from build123d import *

# Parameters (mm, degrees)
FILLET1_R = 5


with BuildPart() as part:
    # Sketch1 → Revolve1 (revolve)
    with BuildSketch(Plane.XY):
        Polygon((16, 0), (9.5, 24.258330249), (9.5, 29.258330249), (18, 37.758330249), (18, 170), (22, 170), (22, 21.6), (20.5, 21.6), (20.5, 18.8), (22, 18.8), (22, 14.8), (20.5, 14.8), (20.5, 12), (22, 12), (22, 4), (19, 4), (19, 0), align=None)
    revolve(axis=Axis((0, 0, 0), (0, 1, 0)))

    # Fillet1
    fillet1_edges = [part.edges().sort_by_distance(p)[0] for p in [
        (-9.5, 29.258330249, 0),
        (-9.5, 24.258330249, 0),
    ]]
    fillet(fillet1_edges, radius=FILLET1_R)


solid = part.part
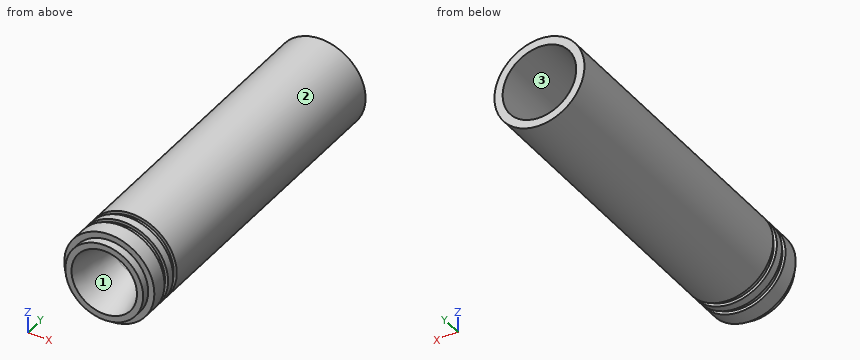
Verification items for the finished model (mm, model axes). Face numbers are marked on the shaded views. Coordinates: 2 decimals unless noted, no trailing zeros. Order: outer loops, then holes, each group sorted by start corner. A loop starts at its lowest first (then second) coordinate and runs counter-clockwise, first axis right, second up. Notation, with made-up numbers: M 88.25,4.25 L 98.25,4.25 A17 cw 98.25,31.25 Z; hole C -24.5,-9.75 d11. An arc over 180 degrees is marked long. One line per item, written item: value. Start each with the question number.
Item 1: Scan lines: probe 1 along Z at (x, y) = (0, 125); probe 2 along Z at (x, y) = (7.5, 161). Record each from-to range of solid material in increasing order.
Item 2: Gauge pin test, flat ends, axial feed: pin 1 (2 mm diameter, centred on x = -16.5, y = 40, fed in from -Z); pin 2 (13 mm diameter, centred on x = 9.5, z = -2.5, fed in from -Y); pin 3 (12 mm diameter, centred on y = 144, z = 15.5, fed in from +X); pin 4 (6 mm diameter, centred on y = 60, z = -7, fed in from -X). Record the tip position at first contact, or that the pin passes through.
Item 3: Mould release check, pull along X, two halves, no side actions. Record for the marked faces 1, 2 and 3: released by +X, released by -X, zero draft, split by the parting line, or undercut.
Item 4: Sectioned sample at A-A (y = 49). Enter the section's corners in (x, z), then the cut area to 3 significant figures.
Conclusion:
1. probe 1: z = -22 to -18, 18 to 22
1. probe 2: z = -20.68 to -16.36, 16.36 to 20.68
2. pin 1: stops at z = -15.61
2. pin 2: stops at y = 0
2. pin 3: stops at x = 19.84
2. pin 4: stops at x = -21.63
3. face 1: undercut
3. face 2: split by the parting line
3. face 3: undercut
4. outline: C 0,0 d44; hole C 0,0 d36
4. area: 503 mm^2
